Build history of the part. All positions in model axes, mm. Face numbers are marked on the shaded views. A direction names the side the tool comes from. Coordinates: 2 decimals unless noted, no trailing zeros. Order: outer loops, then holes, each group sorted by start corner. A loop starts at its lowest first (then second) coordinate and runs counter-clockwise, first axis right, second up. Notation, with made-up numbers: (16.5, 5) - (61.5, 5) arc R24 ccw to (61.5, 19) - close; hole circle Ø10 at (-4, 74). An arc over 180 degrees is marked (long way). Return JSON: item names as keys, results as strings.
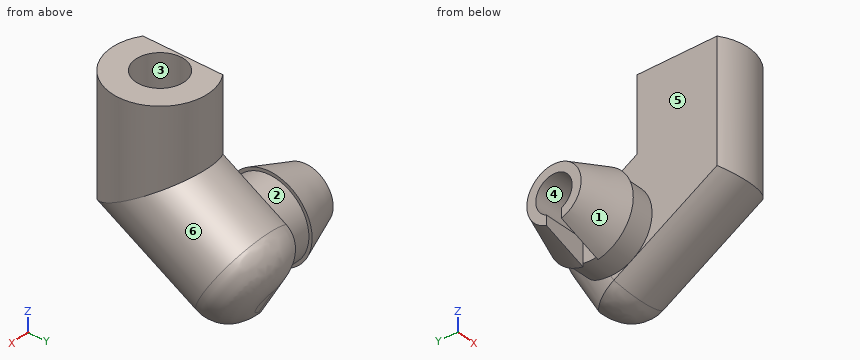
from build123d import *

# Parameters (mm, degrees)
FILLET1_R                       = 1.5
SKETCH3_R                       = 1.125
CUT_EXTRUDE1_DEPTH              = 5.7
SKETCH4_R                       = 1.85
BOSS_EXTRUDE1_DEPTH             = 1.2
BOSS_EXTRUDE1_DIRECTION_2_REACH = 13.17
SKETCH5_R                       = 2
BOSS_EXTRUDE2_DEPTH             = 2
BOSS_EXTRUDE2_TAPER             = 20
SKETCH8_R                       = 0.85
CUT_EXTRUDE2_DEPTH              = 2.4
SKETCH7_W                       = 2
SKETCH7_H                       = 0.7
CUT_EXTRUDE5_DEPTH              = 1.7


with BuildPart() as part:
    # Sweep1: sweep along a path in Sketch2
    with BuildLine(Plane(origin=(0, 0, 0), x_dir=(0, 0, -1), z_dir=(1, 0, 0))) as sweep1_path:
        Line((0, 0), (4.5, 0))
        Line((4.5, 0), (7.5, 5.196152423))
    # Sketch1 → Sweep1 (sweep)
    with BuildSketch(Plane.XY):
        with BuildLine():
            Line((-1.25, 1.870828693), (-1.25, -1.870828693))
            ThreePointArc((-1.25, -1.870828693), (2.25, 0), (-1.25, 1.870828693))
        make_face()
    sweep(path=sweep1_path.line, transition=Transition.RIGHT)

    # Fillet1
    # the kernel refuses this fillet: 1.5 mm, written as the material it takes off along each edge
    with BuildSketch(Plane(origin=(0, 5.196152423, -7.5), x_dir=(-0.9999950652018581, 0.0015707937429397924, 0.0027206945709829077), z_dir=(-0.003141587485879499, -0.4999975326009265, -0.8660211301238867))) as fillet1_piece_1:
        with BuildLine():
            CenterArc((2.25 - FILLET1_R, -FILLET1_R), FILLET1_R, 360, 90)
            Line((2.25 - FILLET1_R, 0), (2.25, 0))
            Line((2.25, 0), (2.25, -FILLET1_R))
        make_face()
    revolve(axis=Axis((0, 5.196152423, -7.5), (0, 0.8660254037844402, -0.49999999999999745)), revolution_arc=359.64, mode=Mode.SUBTRACT)
    with BuildSketch(Plane(origin=(-1.25, 8.006566769, -2.632219561), x_dir=(0, -0.8660254037844399, 0.49999999999999756), z_dir=(0, -0.4999999999999976, -0.86602540378444))) as fillet1_piece_2:
        with BuildLine():
            CenterArc((FILLET1_R, -FILLET1_R), FILLET1_R, 90, 90)
            Line((0, -FILLET1_R), (0, 0))
            Line((0, 0), (FILLET1_R, 0))
        make_face()
    extrude(amount=11.241657387, mode=Mode.SUBTRACT)

    # Sketch3 → Cut-Extrude1 (cut)
    with BuildSketch(Plane.XY):
        Circle(SKETCH3_R)
    extrude(amount=-CUT_EXTRUDE1_DEPTH, mode=Mode.SUBTRACT)

    # Sketch4 → Boss-Extrude1 (add)
    with BuildSketch(Plane.ZY.offset(1.25)):
        with Locations((-6.268038178, 3.020674567)):
            Circle(SKETCH4_R)
    extrude(amount=BOSS_EXTRUDE1_DEPTH)

    # Sketch4 → Boss-Extrude1 direction 2 (add, up to next)
    with BuildSketch(Plane.ZY.offset(1.25), mode=Mode.PRIVATE) as boss_extrude1_direction_2_sk1:
        with Locations((-6.268038178, 3.020674567)):
            Circle(SKETCH4_R)
    boss_extrude1_direction_2_tool1 = extrude(boss_extrude1_direction_2_sk1.sketch, amount=-BOSS_EXTRUDE1_DIRECTION_2_REACH, mode=Mode.PRIVATE) - part.part
    add(boss_extrude1_direction_2_tool1.solids().sort_by_distance((-1.25, 3.020675, -6.268038))[0])

    # Sketch5 → Boss-Extrude2 (add)
    with BuildSketch(Plane.ZY.offset(2.45)):
        with Locations((-6.268038178, 3.020674567)):
            Circle(SKETCH5_R)
    extrude(amount=BOSS_EXTRUDE2_DEPTH, taper=BOSS_EXTRUDE2_TAPER)

    # Sketch8 → Cut-Extrude2 (cut)
    with BuildSketch(Plane.ZY.offset(4.45)):
        with Locations((-6.268038178, 3.020674567)):
            Circle(SKETCH8_R)
    extrude(amount=-CUT_EXTRUDE2_DEPTH, mode=Mode.SUBTRACT)

    # Sketch7 → Cut-Extrude5 (cut, symmetric)
    with BuildSketch(Plane(origin=(0, 0, -8.118038178), x_dir=(-1, 0, 0), z_dir=(0, 0, -1))):
        with Locations((3.45, 3.020674567)):
            Rectangle(SKETCH7_W, SKETCH7_H)
    extrude(amount=CUT_EXTRUDE5_DEPTH, both=True, mode=Mode.SUBTRACT)


solid = part.part
1. Cut at A-A on z = -0.75. Give the cut face in (x, y) (3 decimals).
Check values:
{"outline": "(-1.25, -1.871) arc R2.25 ccw (long way) to (-1.25, 1.871) - close; hole circle Ø2.25 at (0, 0)"}
2. Cut at B-B on x = -3.5. Give the cut face in (y, z).
Check values:
{"outline": "(2.67, -7.85) - (2.67, -7.04) arc R0.85 cw (long way) to (3.37, -7.04) - (3.37, -7.85) arc R1.62 ccw (long way) to start"}
3. Tool access for the marked faces 1, 2 and 3: list every direction of +Z, -Z, +X, -X, +Y, -Y with a clear straight run to the whole face (end or side of a thin tool).
Check values:
{"face 1": "-X", "face 2": "none", "face 3": "+Z"}
4. Probe L1, parallel to X at y = 0.5, z = -2; L2, parallel to Y at x = 0, z = -3.3 (3 decimals); L3, parallel to Y at x = 1, z = -1. List the from-to ranges inside material, lowest first.
Check values:
{"L1": "-1.25 to -1.01, 1.01 to 2.19", "L2": "-2.25 to -1.125, 1.125 to 2.422", "L3": "-2.02 to -0.52, 0.52 to 2.02"}
5. Mould opens along Z. For the marked faces 4, 5 and 6 say: pulls with the +Z half, pulls with the -Z half, needs draft (parallel to the pull), parting line crosses it, or undercut.
Check values:
{"face 4": "undercut", "face 5": "needs draft", "face 6": "parting line crosses it"}
6. Drop flat-ended pins along their axis: pin 1 (2 mm diameter, centred on y = 1.5, z = -5, fed in from -X); pin 2 (2.5 mm diameter, centred on x = 0, y = 0, fed in from -Z); pin 3 (0.7 mm diameter, centred on x = -0.5, y = -0.5, fed in from +Z); pin 4 (2 mm diameter, centred on y = 4, z = -5.5, fed in from +X). Give the stop position or say it passes through.
Check values:
{"pin 1": "x = -4.45", "pin 2": "z = -7.82", "pin 3": "z = -5.7", "pin 4": "x = 2.25"}
